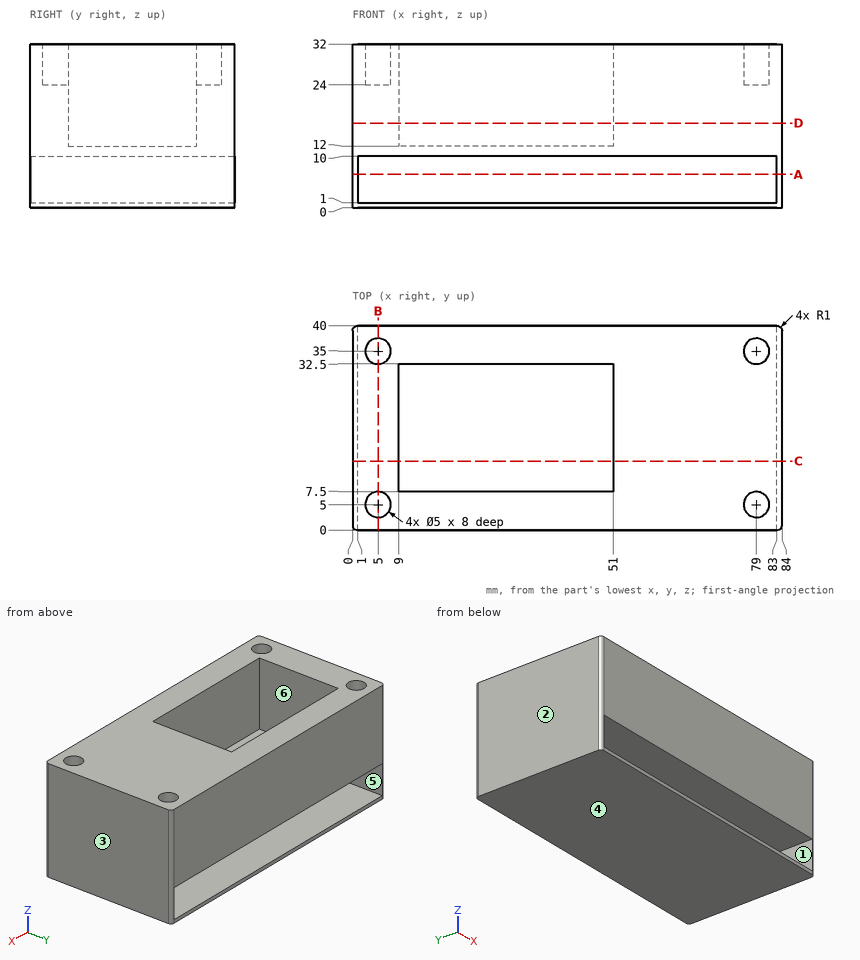
Could you check a few things on this drawing? It's one solid part, dimensions in mm from its lowest x, y, z. A direction names the side the tool comes from. Round coordinates to 2 decimals unless told otherwise and drop trailing zeros. Order: outer loops, then holes, each group sorted by start corner. A loop starts at its lowest first (then second) coordinate and runs counter-clockwise, first axis right, second up. Notation, with made-up numbers: M 70.5,26 L 119.5,26 A24 cw 119.5,51 Z; hole C -9,59 d2. An arc over 180 degrees is marked long. Return JSON: item names as keys, results as strings. Group by question number.
1. If we section it at C-C on y = 13.5: List the corners of the cut face in (x, z) for me, then the cut area to 3 significant figures.
2. If we section it at D-D on z = 16.5: List the corners of the cut face in (x, y) for me.
3. On a 3-axis mill with a long thin cutter (end or side, diameter ignored), from which of +Z, -Z, +X, -X, +Y, -Y can I reach the whole of each face in a straight line? I mean the marked faces 4, 5 and 6. Say none if no direction works.
4. If we mould it in two halves opening along X, with no side actions, what happens to the marked faces 1, 2 and 3? For each: pulls with the +X half, pulls with the -X half, needs draft (parallel to the pull), parting line crosses it, or undercut.
5. I'm going to push flat-ended pins straight in: pin 1 Ø5 at (x, y) = (24.5, 12) entering from +Z; pin 2 Ø4 at (x, y) = (79, 5) entering from +Z. Where does each tip first touch, or does it pass through?
6. If we section it at B-B on x = 5: List the corners of the cut face in (y, z) for me, then the cut area to 3 significant figures.
7. If we section it at A-A on z = 6.5: List the corners of the cut face in (x, y) for me, then the cut area to 3 significant figures.
8. Please list where these lines run through material, in increasing order: probe 1 along X at (y, z) = (35, 30); probe 2 along Y at (x, z) = (5, 27); probe 3 along X at (y, z) = (14.5, 5).
Reply:
{
 "1": {"outline": "M 0,0 L 84,0 L 84,32 L 51,32 L 51,12 L 9,12 L 9,32 L 0,32 Z; hole M 1,1 L 83,1 L 83,10 L 1,10 Z", "area": "1,110 mm^2"},
 "2": {"outline": "M 0,1 A1 ccw 1,0 L 83,0 A1 ccw 84,1 L 84,39 A1 ccw 83,40 L 1,40 A1 ccw 0,39 Z; hole M 9,7.5 L 51,7.5 L 51,32.5 L 9,32.5 Z"},
 "3": {"face 4": "-Z, +X, -X, +Y, -Y", "face 5": "+Y, -Y", "face 6": "+Z"},
 "4": {"face 1": "undercut", "face 2": "pulls with the -X half", "face 3": "pulls with the +X half"},
 "5": {"pin 1": "z = 12", "pin 2": "z = 24"},
 "6": {"outline": "M 0,0 L 40,0 L 40,1 L 0,1 Z; M 0,10 L 40,10 L 40,32 L 37.5,32 L 37.5,24 L 32.5,24 L 32.5,32 L 7.5,32 L 7.5,24 L 2.5,24 L 2.5,32 L 0,32 Z", "area": "840 mm^2"},
 "7": {"outline": "M 0,1 A1 ccw 1,0 L 1,40 A1 ccw 0,39 Z; M 83,0 A1 ccw 84,1 L 84,39 A1 ccw 83,40 Z", "area": "79.1 mm^2"},
 "8": {"probe 1": "0 to 2.5, 7.5 to 76.5, 81.5 to 84", "probe 2": "0 to 2.5, 7.5 to 32.5, 37.5 to 40", "probe 3": "0 to 1, 83 to 84"}
}
